Verification items for this drawing (mm, ordinates from the low corner). A direction names the side the tool comes from. Round coordinates to 2 decimals unless told otherwise and drop trailing zeros. Order: outer loops, then holes, each group sorted by start corner. A loop starts at its lowest first (then second) coordinate and runs counter-clockwise, first axis right, second up. Notation, with made-up numbers: (73, -34) -> (110, -34) arc R24 ccw to (110, -9) -> close; hole circle Ø9 at (36, 68). An arc over 180 degrees is marked (long way). Answer in a Markdown table with one row per item.
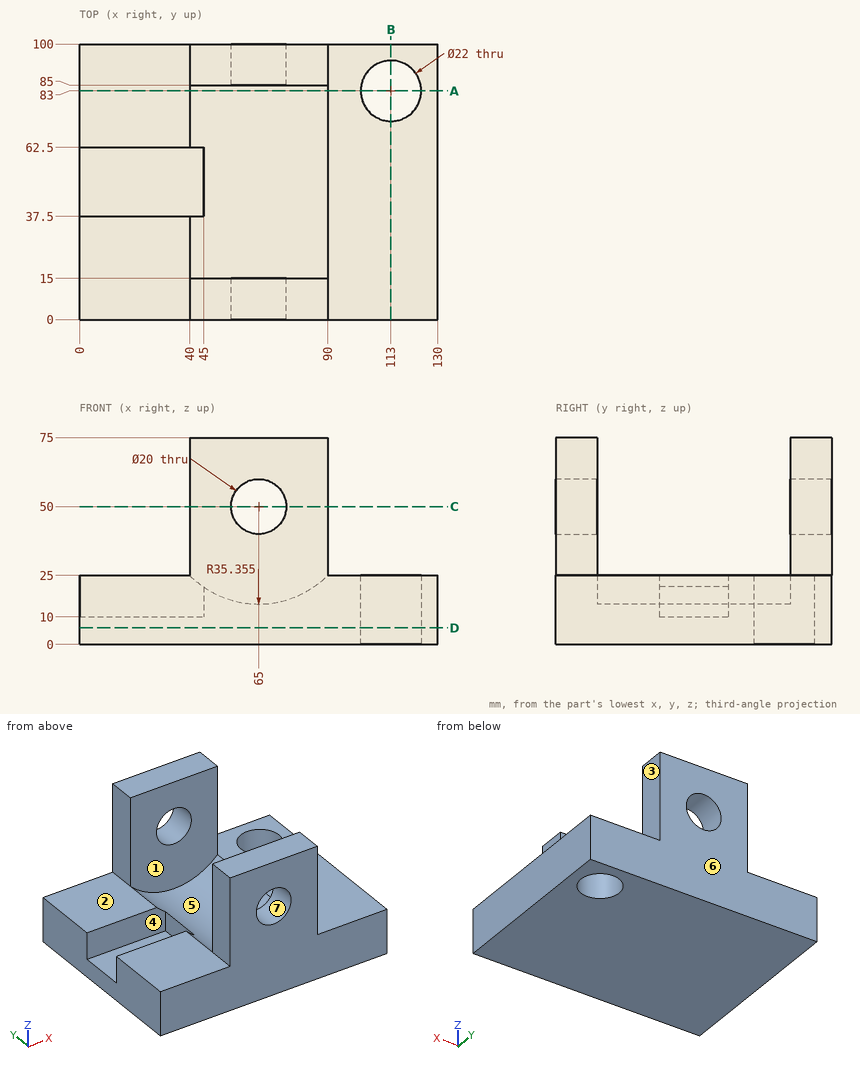
Item 1: Scan lines: line 1 (Y direction, x = 113, z = 11.5); line 2 (X direction, y = 90, z = 50); line 3 (Y direction, x = 18.5, z = 20.5). Record each from-to range of solid material in increasing order. Write a range as [from, to].
Result sheet:
| item | result |
|---|---|
| line 1 | y = [0, 72], [94, 100] |
| line 2 | x = [40, 55], [75, 90] |
| line 3 | y = [0, 37.5], [62.5, 100] |
Item 2: Cross-section at A-A (y = 83). Record the boundary of the cut face in (x, z) (1 decimal).
Result sheet:
| item | result |
|---|---|
| outline | (0, 0) -> (102, 0) -> (102, 25) -> (90, 25) arc R35.4 cw to (40, 25) -> (0, 25) -> close; (124, 0) -> (130, 0) -> (130, 25) -> (124, 25) -> close |
Item 3: Set-up check for the marked faces 1, 2 and 3: record each of +Z, -Z, +X, -X, +Y, -Y from which the full face is reachable in a straight line by a thin tool's end or side.
Result sheet:
| item | result |
|---|---|
| face 1 | +Z |
| face 2 | +Z, -X, +Y, -Y |
| face 3 | +Z, +X, +Y, -Y |
Item 4: Depth check by flat-ended pin: P1, Ø16.5, axis at y = 4, z = 57.5, coming from the -X side; P2, Ø11, axis at x = 29, y = 72, coming from the +Z side; P3, Ø3.5, axis at y = 44, z = 15.5, coming from the -X side; P4, Ø17.5, axis at x = 113, y = 83, coming from the -Z side. Enter the tip coordinate at first touch or a pass-through.
Result sheet:
| item | result |
|---|---|
| P1 | stops at x = 40 |
| P2 | stops at z = 25 |
| P3 | stops at x = 45 |
| P4 | passes through |
Item 5: Cross-section at B-B (x = 113). Record the boundary of the cut face in (y, z).
Result sheet:
| item | result |
|---|---|
| outline | (0, 0) -> (72, 0) -> (72, 25) -> (0, 25) -> close; (94, 0) -> (100, 0) -> (100, 25) -> (94, 25) -> close |
Item 6: Mould release check, pull along Y, two halves, no side actions. Record for the marked faces 4, 5, 6 and 7: pulls with the +Y half, pulls with the -Y half, needs draft (parallel to the pull), parting line crosses it, or undercut.
Result sheet:
| item | result |
|---|---|
| face 4 | undercut |
| face 5 | undercut |
| face 6 | pulls with the +Y half |
| face 7 | needs draft |
Item 7: Cross-section at C-C (z = 50). Record the boundary of the cut face in (x, y).
Result sheet:
| item | result |
|---|---|
| outline | (40, 0) -> (55, 0) -> (55, 15) -> (40, 15) -> close; (40, 85) -> (55, 85) -> (55, 100) -> (40, 100) -> close; (75, 0) -> (90, 0) -> (90, 15) -> (75, 15) -> close; (75, 85) -> (90, 85) -> (90, 100) -> (75, 100) -> close |
Item 8: Cross-section at D-D (z = 6). Record the boundary of the cut face in (x, y), and give its area (3 significant figures).
Result sheet:
| item | result |
|---|---|
| outline | (0, 0) -> (130, 0) -> (130, 100) -> (0, 100) -> close; hole circle Ø22 at (113, 83) |
| area | 12,600 mm^2 |
